Part model, mm, in its own coordinate system. A direction names the side the tool comes from. Round coordinates to 2 decimals unless told otherwise and drop trailing zeros. Write each loop counter-clockwise with the first axis right and the second up, starting at its lowest first coordinate (ties: lowest second). Pieces come first, ordered by that corner, then holes. Notation, with made-up numbers: M 45,52 L 54,52 A29 cw 54,74 Z; hole C -22.75,5.5 d2. An arc over 180 degrees is marked long. Use a Markdown table: item, result. Add a question column.
1) Slice it at C-C on y = 77. Write the cut outline in (x, z).
2) Slice it at A-A on x = 35.75. Write the cut outline in (y, z), plus the area to 3 significant figures.
3) Which spindle directions (+Z, -Z, +X, -X, +Y, -Y) get a long thin tool onto all of the face, cutting with end or side? Do faces 1 (the face through (16, 11, 7)), 2 (the face through (34.12, 69.68, 6.66)). Say none if no direction does.
4) Two-plate mould, pull along X, no slides. Class faces 3 (the face through (35, 56, 0)), 4 (the face through (59.565, 5.423, 7.951)), 5 (the face through (66.6, 104.9, 6.7)), 6 (the face through (5, 105, 7)): released by +X, released by -X, zero draft, split by the parting line, or undercut.
5) Wall check: probe 1 along Z at (x, y) = (55.75, 6); probe 2 along Y at (x, z) = (13, 8.5); probe 3 along Y at (x, z) = (36.5, 7.75). Give the ranges that are in metal, low to high.
6) Slice it at D-D on x = 55.75. Write the cut outline in (y, z).
7) Drop a flat-ended pin along its axis: P1, Ø6.5, axis at x = 54.5, z = 5.5, coming from the -Y side. Give the stop position or say it passes through.
8) Slice it at B-B on z = 6.75. Write the cut outline in (x, y).
```python
from build123d import *

# Parameters (mm, degrees)
SKETCH1_W           = 71.5
SKETCH1_H           = 110
SKETCH1_R           = 7.5
BOSS_EXTRUDE1_DEPTH = 13.5
CHAMFER1_SIZE       = 10
SKETCH2_R           = 4
CUT_EXTRUDE1_DEPTH  = 11


with BuildPart() as part:
    # Sketch1 → Boss-Extrude1 (new body)
    with BuildSketch(Plane.XY):
        with Locations((35.75, 55)):
            Rectangle(SKETCH1_W, SKETCH1_H)
        with Locations((35.75, 77)):
            Circle(SKETCH1_R, mode=Mode.SUBTRACT)
    extrude(amount=BOSS_EXTRUDE1_DEPTH)

    # Chamfer1
    chamfer1_edges = [part.edges().sort_by_distance(p)[0] for p in [
        (0, 110, 6.75),
        (71.5, 110, 6.75),
    ]]
    chamfer(chamfer1_edges, length=CHAMFER1_SIZE)

    # Sketch2 → Cut-Extrude1 (cut)
    with BuildSketch(Plane.XZ):
        with Locations((15.75, 6.75)):
            Circle(SKETCH2_R)
        with Locations((55.75, 6.75)):
            Circle(SKETCH2_R)
    extrude(amount=-CUT_EXTRUDE1_DEPTH, mode=Mode.SUBTRACT)


solid = part.part
```
Entries:
| question | item | result |
|---|---|---|
| 1 | outline | M 0,0 L 28.25,0 L 28.25,13.5 L 0,13.5 Z; M 43.25,0 L 71.5,0 L 71.5,13.5 L 43.25,13.5 Z |
| 2 | outline | M 0,0 L 69.5,0 L 69.5,13.5 L 0,13.5 Z; M 84.5,0 L 110,0 L 110,13.5 L 84.5,13.5 Z |
| 2 | area | 1,280 mm^2 |
| 3 | face 1 | -Y |
| 3 | face 2 | +Z, -Z |
| 4 | face 3 | zero draft |
| 4 | face 4 | undercut |
| 4 | face 5 | released by +X |
| 4 | face 6 | released by -X |
| 5 | probe 1 | z = 0 to 2.75, 10.75 to 13.5 |
| 5 | probe 2 | y = 11 to 110 |
| 5 | probe 3 | y = 0 to 69.54, 84.46 to 110 |
| 6 | outline | M 0,0 L 110,0 L 110,13.5 L 0,13.5 L 0,10.75 L 11,10.75 L 11,2.75 L 0,2.75 Z |
| 7 | P1 | stops at y = 0 |
| 8 | outline | M 0,0 L 11.75,0 L 11.75,11 L 19.75,11 L 19.75,0 L 51.75,0 L 51.75,11 L 59.75,11 L 59.75,0 L 71.5,0 L 71.5,100 L 61.5,110 L 10,110 L 0,100 Z; hole C 35.75,77 d15 |
